Job drawing, mm, ordinate dimensions from the low corner. One solid piece. Give positions to 0.01 mm unless a question says otherwise; leave off trailing zeros. Order: outer loops, then holes, each group sorted by start corner. A loop starts at its lowest first (then second) coordinate and runs counter-clockwise, first axis right, second up. Notation, with made-up numbers: (52, 3.5) - (104, 3.5) arc R17 ccw to (104, 27.5) - close; hole circle Ø8 at (77.5, 18). An arc over 180 degrees is marked (long way). One line per item, written item: value.
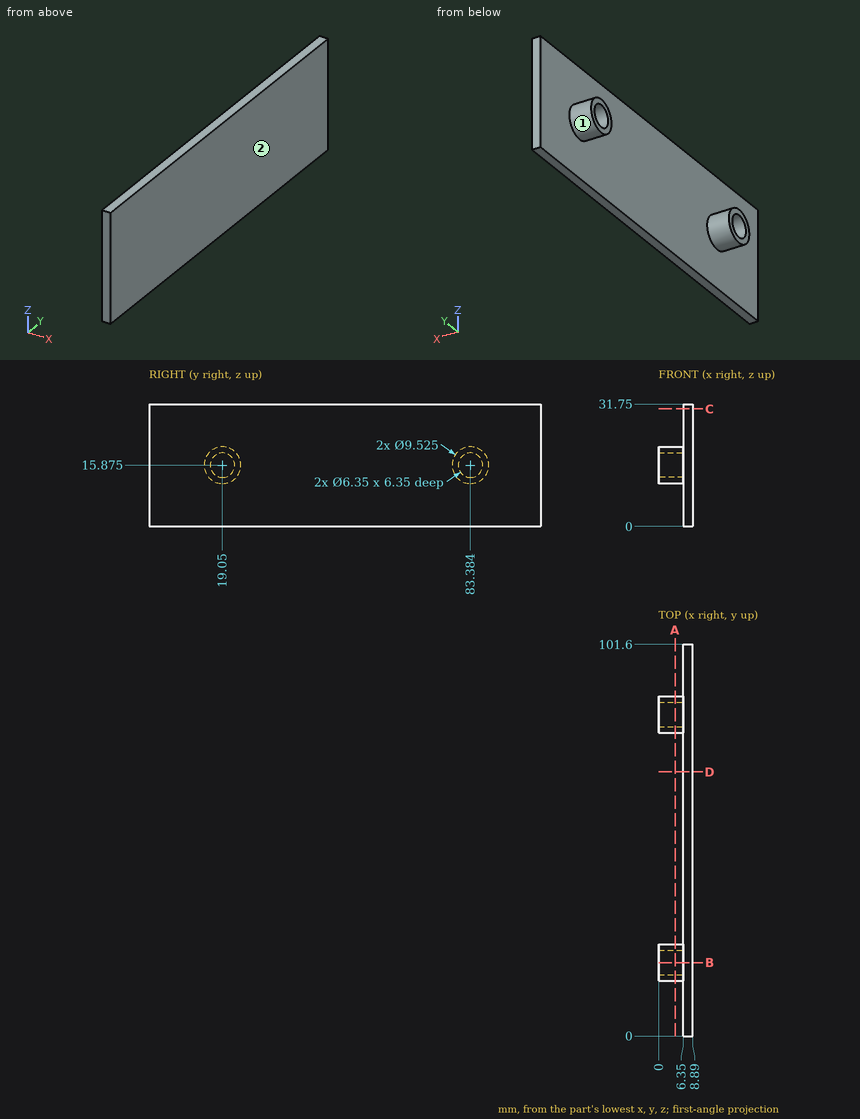
1) Slice it at C-C on z = 30.5. Write the cut outline in (x, y), then the cut area to 3 significant figures.
Answer:
outline: (6.35, 0) - (8.89, 0) - (8.89, 101.6) - (6.35, 101.6) - close
area: 258 mm2
2) Slice it at B-B on y = 19.05. Write the cut outline in (x, z), then the cut area to 3 significant figures.
Answer:
outline: (0, 11.11) - (6.35, 11.11) - (6.35, 0) - (8.89, 0) - (8.89, 31.75) - (6.35, 31.75) - (6.35, 20.64) - (0, 20.64) - (0, 19.05) - (6.35, 19.05) - (6.35, 12.7) - (0, 12.7) - close
area: 101 mm2
3) Drop flat-ended pins along their axis: P1, Ø2, axis at x = 3.5, y = 58.5, coming from the -Z side; P2, Ø5, axis at y = 83, z = 14.5, coming from the -X side; P3, Ø3, axis at y = 36, z = 22.5, coming from the -X side. Give the stop position or say it passes through.
Answer:
P1: passes through
P2: stops at x = 0
P3: stops at x = 6.35
4) Slice it at A-A on x = 4.25. Count the separate pieces of the cut face and the enclosed holes in it.
Answer:
separate pieces: 2
enclosed holes: 2
5) Slice it at D-D on y = 68.5. Write the cut outline in (x, z).
Answer:
outline: (6.35, 0) - (8.89, 0) - (8.89, 31.75) - (6.35, 31.75) - close
6) Two-plate mould, pull along Y, no slides. Class the marked faces 1 and 2: pulls with the +Y half, pulls with the -Y half, needs draft (parallel to the pull), parting line crosses it, or undercut.
Answer:
face 1: undercut
face 2: needs draft
7) Wall check: line 1 along Y through (x, z) = (3, 15) (1 decimal); line 2 along Y through (x, z) = (0.5, 13.5) (1 decimal); line 3 along X through (y, z) = (19.5, 30). Give the ranges that are in metal, low to high. Write a range as [from, to].
Answer:
line 1: y = [14.4, 16], [22.1, 23.7], [78.7, 80.3], [86.4, 88.1]
line 2: y = [14.9, 16.9], [21.2, 23.2], [79.3, 81.3], [85.5, 87.5]
line 3: x = [6.35, 8.89]
